Build history of the part. All positions in model axes, mm. A direction names the side the tool comes from. Give positions to 0.01 mm unless a question says otherwise; leave off trailing zeros. Write each loop counter-clockwise with the first axis right and the second up, starting at its lowest first coordinate (ties: lowest second). Pieces come first, ordered by that corner, then holes. Notation, with made-up numbers: M 82,-2.5 L 141,-2.5 A21 cw 141,4.5 Z; hole C 21.25,-11 d3. An arc over 180 degrees is marked long. Return JSON: item names as keys, results as strings. Group by question number.
Q1. Band-saw the part on C-C, the plane z = 37. Count the separate pieces of the cut face and the enclosed holes in it, then the cut area to 3 significant figures.
Q2. Band-saw the part on B-B, the plane y = 13.5. Give the cut face in (x, z), then the cut area to 3 significant figures.
Q3. Band-saw the part on D-D, the plane x = 29. Give the cut face in (y, z), then the cut area to 3 significant figures.
Q4. Wall check: probe 1 along Y at (x, z) = (0, 56.25); probe 2 along Y at (x, z) = (-0.5, 25.5); probe 3 along Y at (x, z) = (95.5, 43). Give the ranges that are in metal, low to high.
Q5. Tool access for faces 4 (the flat face through (170, 71.042, 31)), 5 (the flat face through (148, 82.07, 31)), 6 (the cylindrical face through (14.198, -74.136, 29.417)): list every direction of +Z, -Z, +X, -X, +Y, -Y with a clear straight run to the whole face (end or side of a thin tool).
Q6. Flat gauge pins, fed straight in: pin 1 Ø6 at (y, z) = (-70.08, 43) entering from +X; pin 2 Ø6.5 at (x, y) = (128.56, 44.81) entering from -Z; pin 3 Ø5 at (x, z) = (182.64, 68) entering from -Y; pin 4 Ø4 at (y, z) = (-70.08, 20) entering from +X. Where does each tip first touch, or does it go through?
Q7. Band-saw the part on A-A, the plane x = 117. Give the cut face in (y, z).
Q8. Pull direction X, two halves, no side cores. Call faces 1 (the flat face through (56, -60, 31)), 2 (the flat face through (-4, 87.07, 31)), 3 (the flat face through (187.642, 79, 31)): +X half, -X half, draft (parallel to the pull), parting line (faces both ways), or undercut.
from build123d import *

# Parameters (mm, degrees)
SKETCH_1_R          = 52.5
EXTRUDE_1_DEPTH     = 63
SKETCH_3_R          = 10
EXTRUDE_3_DEPTH     = 10
EXTRUDE_5_DEPTH     = 57
EXTRUDE_START       = -10
SKETCH_6_R          = 52.5
SKETCH_6_R_2        = 45
EXTRUDE_6_DEPTH     = 10
SKETCH_9_R          = 2.1
CUT_EXTRUDE_1_DEPTH = 10
CUT_EXTRUDE_START   = -10
CUT_EXTRUDE_2_DEPTH = 10
SKETCH_11_R         = 16
CUT_EXTRUDE_3_DEPTH = 8
FILLET_1_R          = 0.5
EXTRUDE_7_DEPTH     = 11.027752017
SKETCH_14_R         = 2.5
CUT_EXTRUDE_5_DEPTH = 135
EXTRUDE_START_2     = 5
SKETCH_16_W         = 47.641975029
SKETCH_16_H         = 63
EXTRUDE_8_DEPTH     = 5
SKETCH_15_R         = 2
CUT_EXTRUDE_7_DEPTH = 14


with BuildPart() as part:
    # 草图1 → 凸台-拉伸1 (new body)
    with BuildSketch(Plane.XY):
        with BuildLine():
            Line((-40.985160522, 43.820276322), (-40.985160522, 71.041954073))
            Line((-40.985160522, 71.041954073), (-77.641975029, 71.041954073))
            Line((-77.641975029, 71.041954073), (-77.641975029, 82.069706091))
            Line((-77.641975029, 82.069706091), (-40.985160522, 82.069706091))
            Line((-40.985160522, 82.069706091), (150.985160522, 82.069706091))
            Line((150.985160522, 82.069706091), (187.641975029, 82.069706091))
            Line((187.641975029, 82.069706091), (187.641975029, 71.041954073))
            Line((187.641975029, 71.041954073), (150.985160522, 71.041954073))
            Line((150.985160522, 71.041954073), (150.985160522, 43.820276322))
            ThreePointArc((150.985160522, 43.820276322), (165.808675756, -22.031607076), (110, -60))
            Line((110, -60), (0, -60))
            ThreePointArc((0, -60), (-55.808675756, -22.031607076), (-40.985160522, 43.820276322))
        make_face()
        Circle(SKETCH_1_R, mode=Mode.SUBTRACT)
        with Locations(Location((110, 0, 0), (0, 0, 180))):
            Circle(SKETCH_1_R, mode=Mode.SUBTRACT)
    extrude(amount=EXTRUDE_1_DEPTH)

    # 草图3 → 凸台-拉伸3 (add)
    with BuildSketch(Plane(origin=(10, 0, 0), x_dir=(0, 0, -1), z_dir=(1, 0, 0))):
        with BuildLine():
            Line((-60, -60), (-60, -90))
            ThreePointArc((-60, -90), (-31.5, -118.5), (-3, -90))
            Line((-3, -90), (-3, -60))
            Line((-3, -60), (-60, -60))
        make_face()
        with Locations((-31.5, -90)):
            Circle(SKETCH_3_R, mode=Mode.SUBTRACT)
    extrude_3 = extrude(amount=EXTRUDE_3_DEPTH)

    # 草图5 → 凸台-拉伸5 (add)
    with BuildSketch(Plane(origin=(0, 0, 3), x_dir=(-1, 0, 0), z_dir=(0, 0, -1))):
        with BuildLine():
            Line((-20, -65), (-20, -60))
            Line((-20, -60), (-25, -60))
            ThreePointArc((-25, -60), (-21.464466094, -61.464466094), (-20, -65))
        make_face()
        with BuildLine():
            Line((-10, -65), (-10, -60))
            Line((-10, -60), (-5, -60))
            ThreePointArc((-5, -60), (-8.535533906, -61.464466094), (-10, -65))
        make_face()
    extrude_5 = extrude(amount=-EXTRUDE_5_DEPTH)

    # 镜向1: 凸台-拉伸3, 凸台-拉伸5 across plane
    add(extrude_3.mirror(Plane(origin=(55, 0, 0), x_dir=(0, 0, 1), z_dir=(1, 0, 0))))
    add(extrude_5.mirror(Plane(origin=(55, 0, 0), x_dir=(0, 0, 1), z_dir=(1, 0, 0))))

    # 草图6 → 凸台-拉伸6 (add)
    # profile 1 of 2: a face of its own
    with BuildSketch(Plane.XY.offset(63).offset(EXTRUDE_START)):
        Circle(SKETCH_6_R)
        Circle(SKETCH_6_R_2, mode=Mode.SUBTRACT)
    # profile 2 of 2: a face of its own
    with BuildSketch(Plane.XY.offset(63).offset(EXTRUDE_START)):
        with Locations(Location((110, 0, 0), (0, 0, 180))):
            Circle(SKETCH_6_R)
        with Locations(Location((110, 0, 0), (0, 0, 180))):
            Circle(SKETCH_6_R_2, mode=Mode.SUBTRACT)
    extrude(amount=EXTRUDE_6_DEPTH)

    # 草图9 → 切除-拉伸1 (cut)
    with BuildSketch(Plane.XY.offset(63)):
        with Locations((65.191842673, 18.56014647)):
            Circle(SKETCH_9_R)
        with Locations((91.43985353, 44.808157327)):
            Circle(SKETCH_9_R)
        with Locations((128.56014647, 44.808157327)):
            Circle(SKETCH_9_R)
        with Locations((154.808157327, 18.56014647)):
            Circle(SKETCH_9_R)
        with Locations((154.808157327, -18.56014647)):
            Circle(SKETCH_9_R)
        with Locations((128.56014647, -44.808157327)):
            Circle(SKETCH_9_R)
        with Locations((91.43985353, -44.808157327)):
            Circle(SKETCH_9_R)
        with Locations((65.191842673, -18.56014647)):
            Circle(SKETCH_9_R)
    cut_extrude_1 = extrude(amount=-CUT_EXTRUDE_1_DEPTH, mode=Mode.SUBTRACT)

    # 镜向2: 切除-拉伸1 across plane
    add(cut_extrude_1.mirror(Plane(origin=(55, 0, 0), x_dir=(0, 0, 1), z_dir=(1, 0, 0))), mode=Mode.SUBTRACT)

    # 草图10 → 切除-拉伸2 (cut)
    with BuildSketch(Plane.XY.offset(63).offset(CUT_EXTRUDE_START)):
        with BuildLine():
            Line((110.985160522, 59.991911611), (110.985160522, 71.041954073))
            Line((110.985160522, 71.041954073), (-0.985160522, 71.041954073))
            Line((-0.985160522, 71.041954073), (-0.985160522, 59.991911611))
            ThreePointArc((-0.985160522, 59.991911611), (32.459672419, 50.461566231), (55, 23.979157617))
            ThreePointArc((55, 23.979157617), (77.540327581, 50.461566231), (110.985160522, 59.991911611))
        make_face()
    cut_extrude_2 = extrude(amount=CUT_EXTRUDE_2_DEPTH, mode=Mode.SUBTRACT)

    # 草图11 → 切除-拉伸3 (cut)
    with BuildSketch(Plane.ZY.offset(-10)):
        with Locations((31.5, -90)):
            Circle(SKETCH_11_R)
    cut_extrude_3 = extrude(amount=-CUT_EXTRUDE_3_DEPTH, mode=Mode.SUBTRACT)

    # 镜向3: 切除-拉伸2 across plane
    add(cut_extrude_2.mirror(Plane.XY.offset(31.5)), mode=Mode.SUBTRACT)

    # 镜向4: 切除-拉伸3 across plane
    add(cut_extrude_3.mirror(Plane(origin=(55, 0, 0), x_dir=(0, 0, 1), z_dir=(1, 0, 0))), mode=Mode.SUBTRACT)

    # 圆角1
    fillet_1_edges = [part.edges().sort_by_distance(p)[0] for p in [
        (10, -90, 15.5),
        (100, -90, 15.5),
    ]]
    fillet(fillet_1_edges, radius=FILLET_1_R)

    # 草图13 → 凸台-拉伸7 (add)
    with BuildSketch(Plane(origin=(0, 82.069706091, 0), x_dir=(1, 0, 0), z_dir=(0, 1, 0))):
        with BuildLine():
            Line((152.641975029, -63), (187.641975029, -63))
            Line((187.641975029, -63), (187.641975029, -68))
            ThreePointArc((187.641975029, -68), (186.177508935, -71.535533906), (182.641975029, -73))
            Line((182.641975029, -73), (162.641975029, -73))
            ThreePointArc((162.641975029, -73), (159.106441123, -71.535533906), (157.641975029, -68))
            ThreePointArc((157.641975029, -68), (156.177508935, -64.464466094), (152.641975029, -63))
        make_face()
        with BuildLine():
            Line((-52.641975029, -73), (-72.641975029, -73))
            ThreePointArc((-72.641975029, -73), (-76.177508935, -71.535533906), (-77.641975029, -68))
            Line((-77.641975029, -68), (-77.641975029, -63))
            Line((-77.641975029, -63), (-42.641975029, -63))
            ThreePointArc((-42.641975029, -63), (-46.177508935, -64.464466094), (-47.641975029, -68))
            ThreePointArc((-47.641975029, -68), (-49.106441123, -71.535533906), (-52.641975029, -73))
        make_face()
        with BuildLine():
            Line((162.641975029, 10), (182.641975029, 10))
            ThreePointArc((182.641975029, 10), (186.177508935, 8.535533906), (187.641975029, 5))
            Line((187.641975029, 5), (187.641975029, 0))
            Line((187.641975029, 0), (152.641975029, 0))
            ThreePointArc((152.641975029, 0), (156.177508935, 1.464466094), (157.641975029, 5))
            ThreePointArc((157.641975029, 5), (159.106441123, 8.535533906), (162.641975029, 10))
        make_face()
        with BuildLine():
            Line((-42.641975029, 0), (-77.641975029, 0))
            Line((-77.641975029, 0), (-77.641975029, 5))
            ThreePointArc((-77.641975029, 5), (-76.177508935, 8.535533906), (-72.641975029, 10))
            Line((-72.641975029, 10), (-52.641975029, 10))
            ThreePointArc((-52.641975029, 10), (-49.106441123, 8.535533906), (-47.641975029, 5))
            ThreePointArc((-47.641975029, 5), (-46.177508935, 1.464466094), (-42.641975029, 0))
        make_face()
        with BuildLine():
            Line((45, -73), (65, -73))
            ThreePointArc((65, -73), (68.535533906, -71.535533906), (70, -68))
            ThreePointArc((70, -68), (71.464466094, -64.464466094), (75, -63))
            Line((75, -63), (35, -63))
            ThreePointArc((35, -63), (38.535533906, -64.464466094), (40, -68))
            ThreePointArc((40, -68), (41.464466094, -71.535533906), (45, -73))
        make_face()
        with BuildLine():
            Line((75, 0), (35, 0))
            ThreePointArc((35, 0), (38.535533906, 1.464466094), (40, 5))
            ThreePointArc((40, 5), (41.464466094, 8.535533906), (45, 10))
            Line((45, 10), (65, 10))
            ThreePointArc((65, 10), (68.535533906, 8.535533906), (70, 5))
            ThreePointArc((70, 5), (71.464466094, 1.464466094), (75, 0))
        make_face()
    extrude(amount=-EXTRUDE_7_DEPTH)

    # 草图14 → 切除-拉伸5 (cut)
    with BuildSketch(Plane.ZY.offset(-10)):
        with Locations((8.5, -90)):
            Circle(SKETCH_14_R)
        with Locations((20, -70.081415713)):
            Circle(SKETCH_14_R)
        with Locations((43, -70.081415713)):
            Circle(SKETCH_14_R)
        with Locations((54.5, -90)):
            Circle(SKETCH_14_R)
        with Locations((43, -109.918584287)):
            Circle(SKETCH_14_R)
        with Locations((20, -109.918584287)):
            Circle(SKETCH_14_R)
    extrude(amount=-CUT_EXTRUDE_5_DEPTH, mode=Mode.SUBTRACT)

    # 草图16 → 凸台-拉伸8 (add)
    with BuildSketch(Plane(origin=(0, 82.069706091, 0), x_dir=(1, 0, 0), z_dir=(0, 1, 0)).offset(EXTRUDE_START_2)):
        with BuildLine():
            Line((-72.641975029, -73), (-52.641975029, -73))
            ThreePointArc((-52.641975029, -73), (-49.106441123, -71.535533906), (-47.641975029, -68))
            Line((-47.641975029, -68), (-47.641975029, 5))
            ThreePointArc((-47.641975029, 5), (-49.106441123, 8.535533906), (-52.641975029, 10))
            Line((-52.641975029, 10), (-72.641975029, 10))
            ThreePointArc((-72.641975029, 10), (-76.177508935, 8.535533906), (-77.641975029, 5))
            Line((-77.641975029, 5), (-77.641975029, -68))
            ThreePointArc((-77.641975029, -68), (-76.177508935, -71.535533906), (-72.641975029, -73))
        make_face()
        with BuildLine():
            Line((40, -68), (40, 5))
            ThreePointArc((40, 5), (41.464466094, 8.535533906), (45, 10))
            Line((45, 10), (65, 10))
            ThreePointArc((65, 10), (68.535533906, 8.535533906), (70, 5))
            Line((70, 5), (70, -68))
            ThreePointArc((70, -68), (68.535533906, -71.535533906), (65, -73))
            Line((65, -73), (45, -73))
            ThreePointArc((45, -73), (41.464466094, -71.535533906), (40, -68))
        make_face()
        with BuildLine():
            Line((162.641975029, 10), (182.641975029, 10))
            ThreePointArc((182.641975029, 10), (186.177508935, 8.535533906), (187.641975029, 5))
            Line((187.641975029, 5), (187.641975029, -68))
            ThreePointArc((187.641975029, -68), (186.177508935, -71.535533906), (182.641975029, -73))
            Line((182.641975029, -73), (162.641975029, -73))
            ThreePointArc((162.641975029, -73), (159.106441123, -71.535533906), (157.641975029, -68))
            Line((157.641975029, -68), (157.641975029, 5))
            ThreePointArc((157.641975029, 5), (159.106441123, 8.535533906), (162.641975029, 10))
        make_face()
        with Locations((113.820987515, -31.5)):
            Rectangle(SKETCH_16_W, SKETCH_16_H)
        with Locations((-3.820987515, -31.5)):
            Rectangle(SKETCH_16_W, SKETCH_16_H)
    extrude(amount=-EXTRUDE_8_DEPTH)

    # 草图15 → 切除-拉伸7 (cut, symmetric)
    with BuildSketch(Plane(origin=(0, 82.069706091, 0), x_dir=(1, 0, 0), z_dir=(0, 1, 0))):
        with Locations(Location((-72.641975029, 5, 0), (0, 0, 270))):
            Circle(SKETCH_15_R)
        with Locations(Location((-52.641975029, 5, 0), (0, 0, 270))):
            Circle(SKETCH_15_R)
        with Locations(Location((45, 5, 0), (0, 0, 270))):
            Circle(SKETCH_15_R)
        with Locations(Location((65, 5, 0), (0, 0, 270))):
            Circle(SKETCH_15_R)
        with Locations(Location((162.641975029, 5, 0), (0, 0, 270))):
            Circle(SKETCH_15_R)
        with Locations(Location((182.641975029, 5, 0), (0, 0, 270))):
            Circle(SKETCH_15_R)
        with Locations(Location((-72.641975029, -68, 0), (0, 0, 270))):
            Circle(SKETCH_15_R)
        with Locations(Location((-52.641975029, -68, 0), (0, 0, 270))):
            Circle(SKETCH_15_R)
        with Locations(Location((45, -68, 0), (0, 0, 270))):
            Circle(SKETCH_15_R)
        with Locations(Location((65, -68, 0), (0, 0, 270))):
            Circle(SKETCH_15_R)
        with Locations(Location((162.641975029, -68, 0), (0, 0, 270))):
            Circle(SKETCH_15_R)
        with Locations(Location((182.641975029, -68, 0), (0, 0, 270))):
            Circle(SKETCH_15_R)
    extrude(amount=CUT_EXTRUDE_7_DEPTH, both=True, mode=Mode.SUBTRACT)


solid = part.part
From the geometry:
{
 "1": {"separate pieces": "3", "enclosed holes": "2", "area": "14,200 mm^2"},
 "2": {"outline": "M -58.46,0 L -50.73,0 L -50.73,53 L -42.93,53 L -42.93,63 L -58.46,63 Z; M 42.93,53 L 50.73,53 L 50.73,0 L 59.27,0 L 59.27,53 L 67.07,53 L 67.07,63 L 42.93,63 Z; M 152.93,53 L 160.73,53 L 160.73,0 L 168.46,0 L 168.46,63 L 152.93,63 Z", "area": "1,820 mm^2"},
 "3": {"outline": "M -60,0 L -43.76,0 L -43.76,53 L -34.41,53 L -34.41,63 L -60,63 Z; M 34.41,53 L 43.76,53 L 43.76,0 L 52.53,0 L 52.53,10 L 71.04,10 L 71.04,0 L 82.07,0 L 82.07,63 L 71.04,63 L 71.04,53 L 52.53,53 L 52.53,63 L 34.41,63 Z", "area": "3,250 mm^2"},
 "4": {"probe 1": "y = -60 to -45, 45 to 60, 71.04 to 87.07", "probe 2": "y = -60 to -52.5, 52.5 to 87.07", "probe 3": "y = -116.08 to -112.42, -107.42 to -101.12, -78.88 to -72.58, -67.58 to -50.46, 50.46 to 87.07"},
 "5": {"face 4": "+Z, -Z, +X", "face 5": "+Z, -Z, +Y", "face 6": "-X"},
 "6": {"pin 1": "stops at x = 100", "pin 2": "stops at z = 53", "pin 3": "stops at y = 71.04", "pin 4": "passes through"},
 "7": {"outline": "M -59.59,0 L -52.03,0 L -52.03,53 L -44.45,53 L -44.45,63 L -59.59,63 Z; M 44.45,53 L 52.03,53 L 52.03,0 L 87.07,0 L 87.07,63 L 44.45,63 Z"},
 "8": {"face 1": "undercut", "face 2": "draft", "face 3": "+X half"}
}
